Source: CAD feature listing. Evaluate the final solid. Frame: model axes, mm. A direction names the side the tool comes from. Give positions to 0.01 mm unless a question says otherwise; leave off trailing zeros. Loops run counter-clockwise (first coordinate to the right, second up) from the corner with the lowest first, then second, coordinate; pieces in that order, holes last. Notation, with made-up numbers: (-10, -38.75) -> (32, -38.75) arc R29 cw to (32, -5.75) -> close; hole circle Ø1 at (51, 87.5). An arc over 180 degrees is marked (long way). Return JSON: item names as keys, results as strings. Group by question number.
(1) Access query for faces 5 (the face through (2, -4, 45)), 6 (the face through (0, 2.5, -34.1)), 7 (the face through (1.18, 5, 1.95)), 8 (the face through (0, 2, 49)). Directions: +Z, -Z, +X, -X, +Y, -Y. A direction counts if a zero-diameter tool reaches every point of the face in a straight line with its end or side. Return the directions, or none.
(2) Pin query (flat end, axial travel): pin 1 (1.5 mm diameter, centred on x = 1, z = 37.5, fed in from +Y); pin 2 (3.5 mm diameter, centred on y = 8.5, z = 49, fed in from -X); pin 3 (0.8 mm diameter, centred on x = 2.5, y = 9.5, fed in from -Z); pin 4 (3 mm diameter, centred on x = 3.5, z = -2.5, fed in from -Y). Return the tip coordinate at first contact, or that it passes through.
(3) Cut plane C-C on z = 49. Return loops of the section in (x, y).
(4) Cut plane B-B on x = -1.25. Return loops of the section in (y, z), then the cut area to 3 significant figures.
(5) Cut plane A-A on z = -3. Return loops of the section in (x, y).
(6) Cut plane D-D on z = 24.5. Return loops of the section in (x, y).
(7) Draft query along X for faces 1 (the face through (-2.1, 2, -16)), 2 (the face through (-5, 2, 4)), 3 (the face through (2, 9, 45)), 4 (the face through (2.1, 2, -16)). Return one class per face: released by +X, released by -X, zero draft, split by the parting line, or undercut.
(8) Ray query, line 1 (Y direction, x = 3, z = 49); line 2 (X direction, y = 4.75, z = -14); line 3 (Z direction, x = 0.5, y = 8.75). Return the intervals inside material, ascending. Write a range as from..to.
```python
from build123d import *

# Parameters (mm, degrees)
BOSS_EXTRUDE1_DEPTH = 5
SKETCH2_W           = 5
SKETCH2_H           = 20
BOSS_EXTRUDE2_DEPTH = 8
SKETCH3_R           = 2.1
CUT_EXTRUDE1_DEPTH  = 8
FILLET2_R           = 2
SKETCH4_W           = 5
SKETCH4_H           = 5
CUT_EXTRUDE2_DEPTH  = 3
FILLET3_R           = 3


with BuildPart() as part:
    # Sketch1 → Boss-Extrude1 (new body)
    with BuildSketch(Plane(origin=(0, 0, 0), x_dir=(1, 0, 0), z_dir=(0, 1, 0))):
        with BuildLine():
            Line((5, 32), (5, 0))
            Line((5, 0), (5, -45))
            Line((5, -45), (-5, -45))
            Line((-5, -45), (-5, 0))
            Line((-5, 0), (-5, 32))
            ThreePointArc((-5, 32), (0, 37), (5, 32))
        make_face()
        with BuildLine():
            Line((2.1, 32), (2.1, 0))
            ThreePointArc((2.1, 0), (0, -2.1), (-2.1, 0))
            Line((-2.1, 0), (-2.1, 32))
            ThreePointArc((-2.1, 32), (0, 34.1), (2.1, 32))
        make_face(mode=Mode.SUBTRACT)
    extrude(amount=BOSS_EXTRUDE1_DEPTH)

    # Sketch2 → Boss-Extrude2 (add)
    with BuildSketch(Plane.XY.offset(45)):
        with Locations((2.5, 2.5)):
            Rectangle(SKETCH2_W, SKETCH2_H)
    extrude(amount=BOSS_EXTRUDE2_DEPTH)

    # Sketch3 → Cut-Extrude1 (cut)
    with BuildSketch(Plane(origin=(5, 0, 0), x_dir=(0, 0, -1), z_dir=(1, 0, 0))):
        with Locations((-49, 8.5)):
            Circle(SKETCH3_R)
        with Locations((-49, -3.5)):
            Circle(SKETCH3_R)
    extrude(amount=-CUT_EXTRUDE1_DEPTH, mode=Mode.SUBTRACT)

    # Fillet2
    fillet2_edges = [part.edges().sort_by_distance(p)[0] for p in [
        (2.5, 12.5, 45),
        (2.5, -7.5, 45),
        (2.5, 12.5, 53),
        (2.5, -7.5, 53),
    ]]
    fillet(fillet2_edges, radius=FILLET2_R)

    # Sketch4 → Cut-Extrude2 (cut)
    with BuildSketch(Plane.XY.offset(45)):
        with Locations((-2.5, 2.5)):
            Rectangle(SKETCH4_W, SKETCH4_H)
    extrude(amount=-CUT_EXTRUDE2_DEPTH, mode=Mode.SUBTRACT)

    # Fillet3
    fillet3_edges = [part.edges().sort_by_distance(p)[0] for p in [
        (2.5, 0, 45),
        (-5, 2.5, 42),
        (2.5, 5, 45),
    ]]
    fillet(fillet3_edges, radius=FILLET3_R)


solid = part.part
```
Answers:
{
 "1": {"face 5": "-Z, +X, -X, -Y", "face 6": "+Y, -Y", "face 7": "-Z, +X, -X, +Y", "face 8": "+Z, -X, +Y, -Y"},
 "2": {"pin 1": "y = 5", "pin 2": "through", "pin 3": "z = 45", "pin 4": "y = 0"},
 "3": {"outline": "(0, -7.5) -> (5, -7.5) -> (5, -5.6) -> (0, -5.6) -> close; (0, -1.4) -> (5, -1.4) -> (5, 6.4) -> (0, 6.4) -> close; (0, 10.6) -> (5, 10.6) -> (5, 12.5) -> (0, 12.5) -> close"},
 "4": {"outline": "(0, -36.84) -> (5, -36.84) -> (5, -33.69) -> (0, -33.69) -> close; (0, 1.69) -> (5, 1.69) -> (5, 42) -> (0, 42) -> close", "area": "217 mm²"},
 "5": {"outline": "(-5, 0) -> (-2.1, 0) -> (-2.1, 5) -> (-5, 5) -> close; (2.1, 0) -> (5, 0) -> (5, 5) -> (2.1, 5) -> close"},
 "6": {"outline": "(-5, 0) -> (5, 0) -> (5, 5) -> (-5, 5) -> close"},
 "7": {"face 1": "undercut", "face 2": "released by -X", "face 3": "zero draft", "face 4": "undercut"},
 "8": {"line 1": "-7.5..-5.6, -1.4..6.4, 10.6..12.5", "line 2": "-5..-2.1, 2.1..5", "line 3": "45..46.91, 51.09..53"}
}
